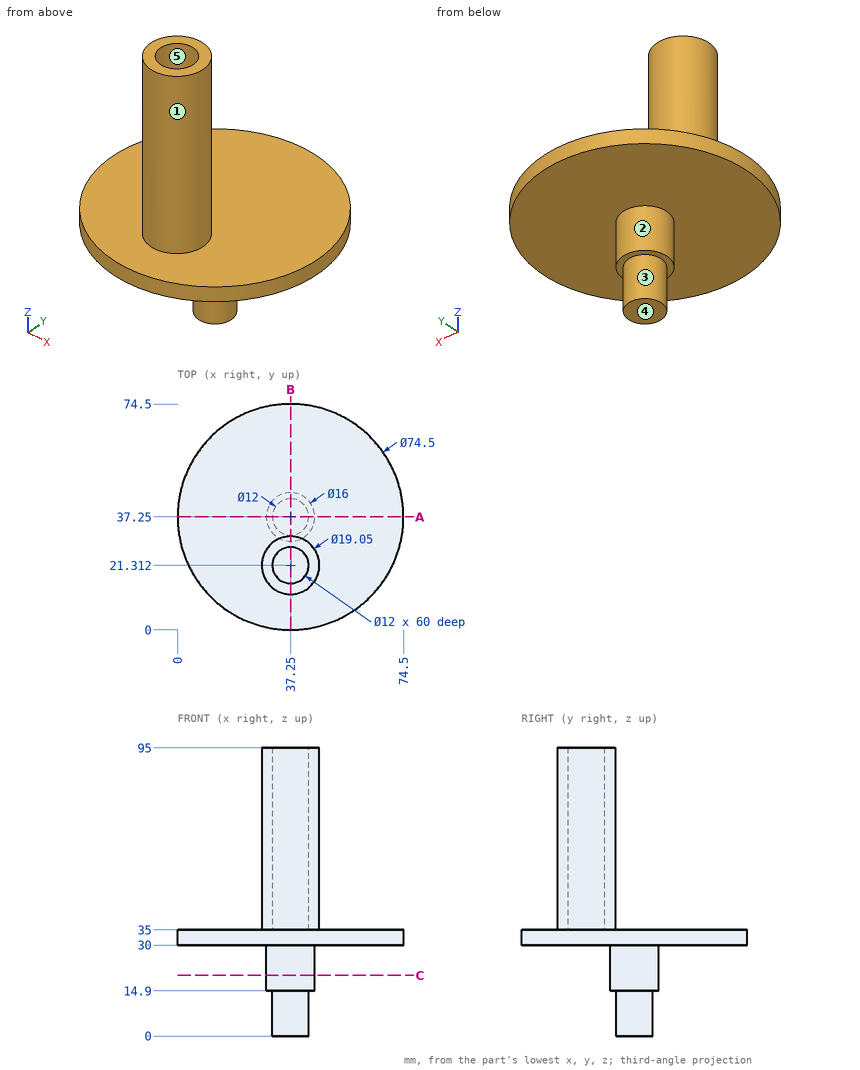
Study the drawing (mm; zero at the part's minimum x, y, z) and answer. A direction names the side the tool comes from. Coordinates: 2 decimals unless noted, no trailing zeros. Write each loop counter-clockwise with the first axis right and the second up, starting at its lowest first coordinate (ties: lowest second). Pieces come first, ordered by that corner, then holes.
Q1. A cutting plane is placed at C-C, the plane z = 20. Give the vertices of the cut face in (x, y).
Q2. A cutting plane is placed at A-A, the plane y = 37.25. Give the vertices of the cut face in (x, z), then the cut area to 3 significant figures.
Q3. A cutting plane is placed at B-B, the plane x = 37.25. Give the vertices of the cut face in (y, z), then the cut area to 3 significant figures.
Q4. Find the intervals of material crossed by line 1 (Y direction, x = 37.25, z = 56); line 2 (Z direction, x = 23.5, y = 64.5); line 3 (X direction, y = 25, z = 84) (1 decimal), in increasing order.
Q5. Each of these flat-tipped pins is pushed along its axis until it touches: pin 1 Ø1 at (x, y) = (65.5, 15.5) entering from -Z; pin 2 Ø6 at (x, y) = (37.5, 20) entering from +Z; pin 3 Ø10 at (y, z) = (56, 32.5) entering from +X. Where does it stop, or does it pass through?
Q6. Determine the mould class of the marked faces 3, 4 and 5 for opening direction X: released by +X, released by -X, zero draft, split by the parting line, or undercut.
Q7. Which of the six approach directions +Z, -Z, +X, -X, +Y, -Y give full straight-line access (tool end or side, diameter ignored) to the marked faces 1 and 2?
Findings below:
1. outline: circle Ø16 at (37.25, 37.25)
2. outline: (0, 30) - (29.25, 30) - (29.25, 14.9) - (31.25, 14.9) - (31.25, 0) - (43.25, 0) - (43.25, 14.9) - (45.25, 14.9) - (45.25, 30) - (74.5, 30) - (74.5, 35) - (0, 35) - close
2. area: 793 mm2
3. outline: (0, 30) - (29.25, 30) - (29.25, 14.9) - (31.25, 14.9) - (31.25, 0) - (43.25, 0) - (43.25, 14.9) - (45.25, 14.9) - (45.25, 30) - (74.5, 30) - (74.5, 35) - (30.84, 35) - (30.84, 95) - (27.31, 95) - (27.31, 35) - (15.31, 35) - (15.31, 95) - (11.79, 95) - (11.79, 35) - (0, 35) - close
3. area: 1,220 mm2
4. line 1: y = 11.79 to 15.31, 27.31 to 30.84
4. line 2: z = 30 to 35
4. line 3: x = 28.5 to 32.5, 42 to 46
5. pin 1: stops at z = 30
5. pin 2: stops at z = 35
5. pin 3: stops at x = 71.87
6. face 3: split by the parting line
6. face 4: zero draft
6. face 5: undercut
7. face 1: +Z
7. face 2: -Z
